Part model, mm, in its own coordinate system. A direction names the side the tool comes from. Give positions to 0.01 mm unless a question says otherwise; leave off trailing zeros. Write each loop counter-clockwise with the first axis right and the second up, starting at its lowest first coordinate (ties: lowest second). Pieces come first, ordered by that corner, then holes. Notation, with made-up numbers: M 68.25,26.25 L 95.25,26.25 A11 ccw 95.25,36.25 Z; hole C 3.25,44.25 d10. An arc over 180 degrees is marked long. Use CSV: the item, a comma, the result in double quotes. Start each with the question number.
1. Drill centre lines: line 1 along X through (y, z) = (16.5, 12.25); line 2 along X through (y, z) = (0, 7); line 3 along X through (y, z) = (0, 4.5). Where is each one in solid material? Low to high. Write a range as from..to.
2. Mould opens along X. For faces 1 (the face through (28, 0, 12.7)), 2 (the face through (-36, 0, 6.35)), 3 (the face through (-50.8, 0, 6)), 4 (the face through (50.8, 0, 6)) say: pulls with the +X half, pulls with the -X half, needs draft (parallel to the pull), parting line crosses it, or undercut.
3. Band-saw the part on A-A, the plane y = 0. List the corners of the cut face in (x, z), then the cut area to 3 significant figures.
4. Band-saw the part on D-D, the plane y = -9. List the corners of the cut face in (x, z), then the cut area to 3 significant figures.
5. Drop flat-ended pins along their axis: pin 1 Ø12 at (x, y) = (2.5, 0.5) entering from -Z; pin 2 Ø4 at (x, y) = (-1.5, 17) entering from +Z. Give the stop position or say it passes through.
6. Band-saw the part on C-C, the plane z = 2.5. List the corners of the cut face in (x, y), then the cut area to 3 significant figures.
7. 3-axis set-ups, long thin cutter, end or side, ignore diameter. For faces 5 (the face through (-45, 0, 12.7)), 6 (the face through (-6.35, 18, 10)): which of +Z, -Z, +X, -X, +Y, -Y reach the whole face in a straight line?
8. Band-saw the part on B-B, the plane x = 0. List the corners of the cut face in (y, z).
from build123d import *

# Parameters (mm, degrees)
F0_W     = 101.6
F0_H     = 50.8
F0_R     = 12.7
F1_DEPTH = 12.7
F2_W     = 6.35
F2_H     = 50.8
F3_DEPTH = 6.35


with BuildPart() as f1:
    # F0 (on Top) → F1 (new body)
    with BuildSketch(Plane.XY):
        Rectangle(F0_W, F0_H)
        Circle(F0_R, mode=Mode.SUBTRACT)
    extrude(amount=F1_DEPTH)

    # F2 (on face) → F3 (cut)
    with BuildSketch(Plane.XY.offset(12.7)):
        with Locations((-36.4539266646, 0)):
            Rectangle(F2_W, F2_H)
        with BuildLine():
            Line((-6.35, -10.9985226281), (-6.35, -25.4))
            Line((-6.35, -25.4), (6.35, -25.4))
            Line((6.35, -25.4), (6.35, -10.9985226281))
            ThreePointArc((6.35, -10.9985226281), (0, -12.7), (-6.35, -10.9985226281))
        make_face()
        with BuildLine():
            Line((6.35, 25.4), (-6.35, 25.4))
            Line((-6.35, 25.4), (-6.35, 10.9985226281))
            ThreePointArc((-6.35, 10.9985226281), (0, 12.7), (6.35, 10.9985226281))
            Line((6.35, 10.9985226281), (6.35, 25.4))
        make_face()
    extrude(amount=-F3_DEPTH, mode=Mode.SUBTRACT)


solid = f1.part
Output:
1,line 1,"x = -50.8..-39.63, -33.28..-6.35, 6.35..50.8"
1,line 2,"x = -50.8..-39.63, -33.28..-12.7, 12.7..50.8"
1,line 3,"x = -50.8..-12.7, 12.7..50.8"
2,face 1,"needs draft"
2,face 2,"undercut"
2,face 3,"pulls with the -X half"
2,face 4,"pulls with the +X half"
3,outline,"M -50.8,0 L -12.7,0 L -12.7,12.7 L -33.28,12.7 L -33.28,6.35 L -39.63,6.35 L -39.63,12.7 L -50.8,12.7 Z; M 12.7,0 L 50.8,0 L 50.8,12.7 L 12.7,12.7 Z"
3,area,"927 mm²"
4,outline,"M -50.8,0 L -8.96,0 L -8.96,12.7 L -33.28,12.7 L -33.28,6.35 L -39.63,6.35 L -39.63,12.7 L -50.8,12.7 Z; M 8.96,0 L 50.8,0 L 50.8,12.7 L 8.96,12.7 Z"
4,area,"1,020 mm²"
5,pin 1,"passes through"
5,pin 2,"stops at z = 6.35"
6,outline,"M -50.8,-25.4 L 50.8,-25.4 L 50.8,25.4 L -50.8,25.4 Z; hole C 0,0 d25.4"
6,area,"4,650 mm²"
7,face 5,"+Z, +X, -X, +Y, -Y"
7,face 6,"+Z, +Y, -Y"
8,outline,"M -25.4,0 L -12.7,0 L -12.7,6.35 L -25.4,6.35 Z; M 12.7,0 L 25.4,0 L 25.4,6.35 L 12.7,6.35 Z"
